from build123d import *

# Parameters (mm, degrees)
ESBO_O1_W                 = 9.525
ESBO_O1_H                 = 25.4
RESSALTO_EXTRUS_O1_DEPTH  = 210
FILETE1_R                 = 1
CORTE_EXTRUS_O1_START     = -9.525
CORTE_EXTRUS_O1_DEPTH     = 9.525
FURO_ROSCADO_DE_M6X1_01_D = 5


# Read off the part's stored shape, not the designer's step: Corte-extrusão1
with BuildPart() as part:
    # Esboço1 → Ressalto-extrusão1 (new, symmetric)
    with BuildSketch(Plane.XY):
        Rectangle(ESBO_O1_W, ESBO_O1_H)
    extrude(amount=RESSALTO_EXTRUS_O1_DEPTH, both=True)

    # Filete1
    filete1_edges = [part.edges().sort_by_distance(p)[0] for p in [
        (4.7625, -12.7, 0),
        (-4.7625, -12.7, 0),
        (-4.7625, 12.7, 0),
        (4.7625, 12.7, 0),
    ]]
    fillet(filete1_edges, radius=FILETE1_R)

    # Corte-extrusão1 outline → Corte-extrusão1 (cut)
    with BuildSketch(Plane.ZY.offset(4.7625).offset(CORTE_EXTRUS_O1_START)):
        Polygon((118.94, 12.7), (122.111992176, -12.7), (210, -12.7), (210, 12.7), align=None)
        Polygon((-210, -12.7), (-122.111992176, -12.7), (-118.94, 12.7), (-210, 12.7), align=None)
    extrude(amount=CORTE_EXTRUS_O1_DEPTH, mode=Mode.SUBTRACT)

    # Furo roscado de M6x1.01 (through all)
    with Locations(Plane.ZY.offset(4.7625)):
        with Locations((-100, 0), (100, 0)):
            Hole(FURO_ROSCADO_DE_M6X1_01_D / 2)


solid = part.part
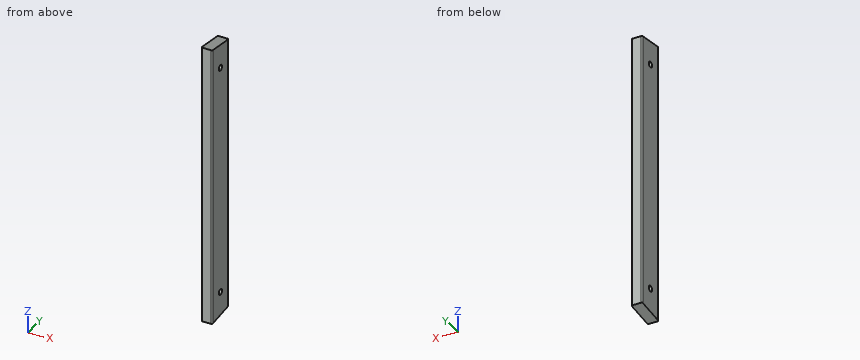
Source: CAD feature listing. Evaluate the final solid. Frame: model axes, mm. Round coordinates to 2 decimals unless told otherwise and drop trailing zeros. Loops run counter-clockwise (first coordinate to the right, second up) from the corner with the lowest first, then second, coordinate; pieces in that order, holes last. Notation, with made-up numbers: (-21.5, -14.5) - (18.5, -14.5) arc R28 ccw to (18.5, 12.5) - close; hole circle Ø8 at (73.5, 14.25). An arc over 180 degrees is marked (long way). Write item = value, one per line. Start each with the question number.
Item 1: Section query B-B on x = -1.5. Output: boundary loops of the cut face in (y, z).
Item 2: Section query C-C on y = 0. Output: boundary loops of the cut face in (x, z).
Item 3: Material intervals for line 1 (Y direction, x = 1, z = 100); line 2 (Z direction, x = -3.5, y = -1.25); line 3 (Y direction, x = 3.5, z = -101), sorted ascending.
Item 4: Section query A-A on z = -100. Output: boundary loops of the cut face in (x, y), plus the area to 3 significant figures.
Item 5: First-contact query: pin 1 Ø5 at (x, y) = (2, 8) entering from +Z; pin 2 Ø8 at (y, z) = (0, 100) entering from -X; pin 3 Ø2 at (x, y) = (0, 4) entering from +Z. Flat tips, straight axial feed; report the tip coordinate or a pass-through.
Results list:
q1.outline = (-12.7, -122.11) - (12.7, -118.94) - (12.7, 118.94) - (-12.7, 122.11) - close; hole circle Ø5 at (0, -100); hole circle Ø5 at (0, 100)
q2.outline = (-4.76, -120.53) - (4.76, -120.53) - (4.76, -102.5) - (-4.76, -102.5) - close; (-4.76, -97.5) - (4.76, -97.5) - (4.76, 97.5) - (-4.76, 97.5) - close; (-4.76, 102.5) - (4.76, 102.5) - (4.76, 120.53) - (-4.76, 120.53) - close
q3.line_1 = -12.7 to -2.5, 2.5 to 12.7
q3.line_2 = -120.68 to -102.17, -97.83 to 97.83, 102.17 to 120.68
q3.line_3 = -12.7 to -2.29, 2.29 to 12.7
q4.outline = (-4.76, -11.7) arc R1 ccw to (-3.76, -12.7) - (3.76, -12.7) arc R1 ccw to (4.76, -11.7) - (4.76, -2.5) - (-4.76, -2.5) - close; (-4.76, 2.5) - (4.76, 2.5) - (4.76, 11.7) arc R1 ccw to (3.76, 12.7) - (-3.76, 12.7) arc R1 ccw to (-4.76, 11.7) - close
q4.area = 193 mm²
q5.pin_1 = 119.84
q5.pin_2 = -4.76
q5.pin_3 = 120.15
